Could you check a few things on this model? Use its own coordinates, in mm. Face numbers are marked on the shaded views. A direction names the side the tool comes from. Coordinates: 2 decimals unless noted, no trailing zeros. Write each loop counter-clockwise with the first axis right and the second up, starting at its lowest first coordinate (ties: lowest second). Pieces come first, ordered by that corner, then holes.
```python
from build123d import *

# Parameters (mm, degrees)
BOSS_EXTRUDE1_DEPTH      = 6.35
BOSS_EXTRUDE2_DEPTH      = 12.192
BOSS_EXTRUDE3_REACH      = 63.797
CUT_EXTRUDE1_DEPTH       = 3.175
CUT_EXTRUDE2_DEPTH       = 3.175
F_8_0_8_DIAMETER_HOLE1_D = 8
HOLE1_D                  = 6.35
CHAMFER1_SIZE            = 3.256138018
CHAMFER2_SIZE            = 2.651435284
FILLET1_R                = 0.762
FILLET2_R                = 17.78


with BuildPart() as part:
    # Sketch1 → Boss-Extrude1 (new body)
    with BuildSketch(Plane.XY):
        with BuildLine():
            Line((-25.876615107, -6.130991244), (-6.855570788, -16.51429077))
            ThreePointArc((-6.855570788, -16.51429077), (-12.797339629, -25.300522195), (-4.835774214, -32.308799856))
            Line((-4.835774214, -32.308799856), (5.019425786, -32.308799856))
            ThreePointArc((5.019425786, -32.308799856), (12.97831912, -25.32120391), (7.079560008, -16.524890981))
            Line((7.079560008, -16.524890981), (44.341655967, -6.756691298))
            ThreePointArc((44.341655967, -6.756691298), (49.5554, 0), (44.341655967, 6.756691298))
            Line((44.341655967, 6.756691298), (-2.321508902, 18.989366367))
            Line((-2.321508902, 18.989366367), (-25.876615107, 6.130991244))
            ThreePointArc((-25.876615107, 6.130991244), (-29.5148, 0), (-25.876615107, -6.130991244))
        make_face()
    extrude(amount=-BOSS_EXTRUDE1_DEPTH)

    # Sketch2 → Boss-Extrude2 (add)
    with BuildSketch(Plane(origin=(0, 0, -6.35), x_dir=(-1, 0, 0), z_dir=(0, 0, -1))):
        with BuildLine():
            Line((4.835774214, -34.848799856), (-5.019425786, -34.848799856))
            ThreePointArc((-5.019425786, -34.848799856), (-14.222989868, -29.47308547), (-14.061825786, -18.815791108))
            Line((-14.061825786, -18.815791108), (-14.061825783, -4.219323287))
            ThreePointArc((-14.061825783, -4.219323287), (-12.289675842, 8.031282652), (-1.781242501, 14.572741966))
            Line((-1.781242501, 14.572741966), (-1.778349168, 14.573095333))
            ThreePointArc((-1.778349168, 14.573095333), (11.415932367, 9.231149524), (13.878174214, -4.788936617))
            Line((13.878174214, -4.788936617), (13.878174214, -18.815791108))
            ThreePointArc((13.878174214, -18.815791108), (14.039338296, -29.47308547), (4.835774214, -34.848799856))
        make_face()
    extrude(amount=BOSS_EXTRUDE2_DEPTH)

    # Boss-Extrude3: up to this plane
    boss_extrude3_end = Plane(origin=(5.084615624, 0, -17.49223415), z_dir=(0.2791253467698281, 0, -0.9602546749642114))
    # Sketch4 → Boss-Extrude3 (add, up to the surface)
    with BuildSketch(Plane(origin=(0, 0, -6.35), x_dir=(-1, 0, 0), z_dir=(0, 0, -1)), mode=Mode.PRIVATE) as boss_extrude3_sk1:
        with BuildLine():
            Line((-36.092721498, 7.827214142), (-9.663817118, 11.052070939))
            ThreePointArc((-9.663817118, 11.052070939), (-14.107813549, 4.062909083), (-14.061825786, -4.219323276))
            Line((-14.061825786, -4.219323276), (-14.061825786, -10.512648454))
            Line((-14.061825786, -10.512648454), (-36.084688558, -7.820559257))
            ThreePointArc((-36.084688558, -7.820559257), (-32.410401339, 0.005215736), (-36.092721498, 7.827214142))
        make_face()
    boss_extrude3_tool1 = split(extrude(boss_extrude3_sk1.sketch, amount=BOSS_EXTRUDE3_REACH, mode=Mode.PRIVATE), bisect_by=boss_extrude3_end, keep=Keep.BOTH, mode=Mode.PRIVATE)
    add(boss_extrude3_tool1.solids().sort_by_distance((23.208362, 0.258221, -6.35))[0])

    # Sketch5 → Cut-Extrude1 (cut)
    with BuildSketch(Plane.XY):
        with BuildLine():
            Line((17.683274588, 1.852079867), (37.689391665, 1.852079867))
            ThreePointArc((37.689391665, 1.852079867), (39.677118992, 3.014104647), (38.515094212, 5.001831974))
            Line((38.515094212, 5.001831974), (15.636334606, 10.999462718))
            ThreePointArc((15.636334606, 10.999462718), (14.82307645, 10.705321164), (14.808458463, 9.840627925))
            ThreePointArc((14.808458463, 9.840627925), (16.729686315, 6.020464751), (17.683274588, 1.852079867))
        make_face()
    extrude(amount=-CUT_EXTRUDE1_DEPTH, mode=Mode.SUBTRACT)

    # Sketch6 → Cut-Extrude2 (cut)
    with BuildSketch(Plane.XY):
        with BuildLine():
            Line((15.636334606, -10.999462718), (38.515094212, -5.001831974))
            ThreePointArc((38.515094212, -5.001831974), (39.677118992, -3.014104647), (37.689391665, -1.852079867))
            Line((37.689391665, -1.852079867), (17.683274588, -1.852079867))
            ThreePointArc((17.683274588, -1.852079867), (16.729686315, -6.020464751), (14.808458463, -9.840627925))
            ThreePointArc((14.808458463, -9.840627925), (14.82307645, -10.705321164), (15.636334606, -10.999462718))
        make_face()
    extrude(amount=-CUT_EXTRUDE2_DEPTH, mode=Mode.SUBTRACT)

    # Sketch7 → Cut-Revolve1 (revolve, cut)
    with BuildSketch(Plane(origin=(0, 0, 0), x_dir=(1, 0, 0), z_dir=(0, 1, 0))):
        Polygon((10.795, 9.9822), (0, 9.9822), (0, 0), (15.24, 0), (15.24, 1.905), (13.9827, 1.905), (13.9827, 3.81), (10.795, 3.81), align=None)
    revolve(axis=Axis((0, 0, -9.9822), (0, 0, 1)), mode=Mode.SUBTRACT)

    # Ø8.0 (8) Diameter Hole1 (through all)
    with Locations(Plane.XY):
        with Locations((0.034636225, -24.282399856)):
            Hole(F_8_0_8_DIAMETER_HOLE1_D / 2)

    # Hole1 (through all)
    with Locations(Plane(origin=(0, 0, -6.35), x_dir=(-1, 0, 0), z_dir=(0, 0, -1))):
        with Locations((-42.5704, 0), (22.5298, 0)):
            Hole(HOLE1_D / 2)

    # Chamfer1
    # the kernel refuses this chamfer: 3.256138018, 2.953062062 mm, written as the material it adds along each edge
    with BuildSketch(Plane(origin=(-6.855570788, -16.51429077, 0), x_dir=(-0.8777367565349716, 0.4791431792559171, 0), z_dir=(0, 0, -1))) as chamfer1_piece_1:
        with BuildLine():
            Line((CHAMFER1_SIZE, 0), (1.840697413, -2.592929003))
            ThreePointArc((1.840697413, -2.592929003), (1.066981917, -1.228355945), (0, 0))
            Line((0, 0), (CHAMFER1_SIZE, 0))
        make_face()
    extrude(amount=14.651282068)

    # Chamfer2
    # the kernel refuses this chamfer: 2.653671842, 2.651435284 mm, written as the material it adds along each edge
    with BuildSketch(Plane(origin=(7.079560008, -16.524890981, 0), x_dir=(0.9060971467141865, -0.4230696877778058, 0), z_dir=(0, 0, -1))) as chamfer2_piece_1:
        with BuildLine():
            Line((2.830570234, 0), (CHAMFER2_SIZE * 0.769198854398, -CHAMFER2_SIZE * 0.639009485396))
            Line((CHAMFER2_SIZE * 0.769198854398, -CHAMFER2_SIZE * 0.639009485396), (0, 0))
            ThreePointArc((0, 0), (1.438235904, -0.125730188), (2.830570234, 0))
        make_face()
    extrude(amount=13.542714548)

    # Fillet1
    fillet1_edges = [part.edges().sort_by_distance(p)[0] for p in [
        (17.683274588, 1.852079867, -1.5875),
        (17.683274588, -1.852079867, -1.5875),
    ]]
    fillet(fillet1_edges, radius=FILLET1_R)

    # Fillet2
    fillet2_edges = [part.edges().sort_by_distance(p)[0] for p in [
        (-2.321508902, 18.989366367, -3.175),
    ]]
    fillet(fillet2_edges, radius=FILLET2_R)


solid = part.part
```
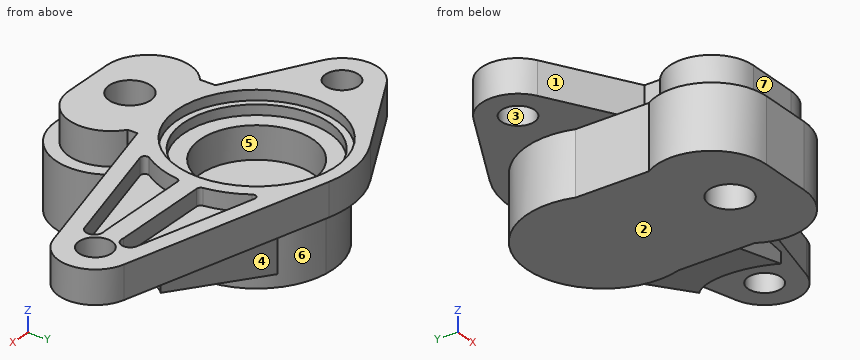
Item 1: If I drill on line 1 along Y through (x, z) = (0, -3.1); line 2 along Z through (x, y) = (2.5, -14.5) (3 decimals); line 3 along X through (y, z) = (-14.5, -13.5), over which ranges is the centre line in solid material (lowest first)?
Item 2: Which directions (+Z, -Z, +X, -X, +Y, -Y) give clear straight access to the entire face, cutting with the end or side of a thin tool? Please do the marked faces 5, 6 and 7.
Item 3: I want a section at B-B, the plane y = 0. Count the separate pieces of the cut face and the enclosed holes in it, then the cut area to 3 significant figures.
Item 4: I want a section at A-A, the plane x = -21. List the corners of the cut face in (y, z) for me, then the cut area to 3 significant figures.
Item 5: If we mould it in two halves opening along Y, with no side actions, what happens to the marked faces 1, 2, 3 and 4? For each: released by +Y, released by -Y, zero draft, split by the parting line, or undercut.
Item 6: Will these pins go through, and if not, where does the flat tip stop? pin 1 Ø10 at (y, z) = (-11, -11.5) entering from -X; pin 2 Ø1 at (x, z) = (20.5, -12.5) entering from +Y; pin 3 Ø6 at (x, z) = (9.5, -10.5) entering from +Y; pin 4 Ø4 at (x, y) = (42.57, 0) entering from -Z.
Item 7: I want a section at D-D, the plane x = 0. List the corners of the cut face in (y, z) for me (3 decimals).
Taken from the geometry:
1. line 1: y = -32.31 to -28.28, -20.28 to -13.98, 13.98 to 17.78
1. line 2: z = -18.542 to -1.905
1. line 3: x = -13.88 to 14.06
2. face 5: +Z
2. face 6: -Z, +X
2. face 7: +Z, +X, -X, -Y
3. separate pieces: 3
3. enclosed holes: 0
3. area: 637 mm2
4. outline: (-8.79, -6.35) - (-2.78, -6.35) - (-2.78, 0) - (-8.79, 0) - close; (2.78, -6.35) - (8.79, -6.35) - (8.79, 0) - (2.78, 0) - close
4. area: 76.3 mm2
5. face 1: undercut
5. face 2: zero draft
5. face 3: undercut
5. face 4: released by +Y
6. pin 1: stops at x = -13.88
6. pin 2: stops at y = 9.79
6. pin 3: stops at y = 13.16
6. pin 4: passes through
7. outline: (-34.849, -18.542) - (-28.282, -18.542) - (-28.282, 0) - (-32.309, 0) - (-32.309, -6.35) - (-34.849, -6.35) - close; (-20.283, -18.542) - (14.681, -18.542) - (14.681, -6.35) - (17.78, -6.35) - (17.78, 0) - (15.24, 0) - (15.24, -1.905) - (13.983, -1.905) - (13.983, -3.81) - (10.795, -3.81) - (10.795, -9.982) - (-10.795, -9.982) - (-10.795, -3.81) - (-13.983, -3.81) - (-13.983, -1.905) - (-15.24, -1.905) - (-15.24, 0) - (-20.283, 0) - close
